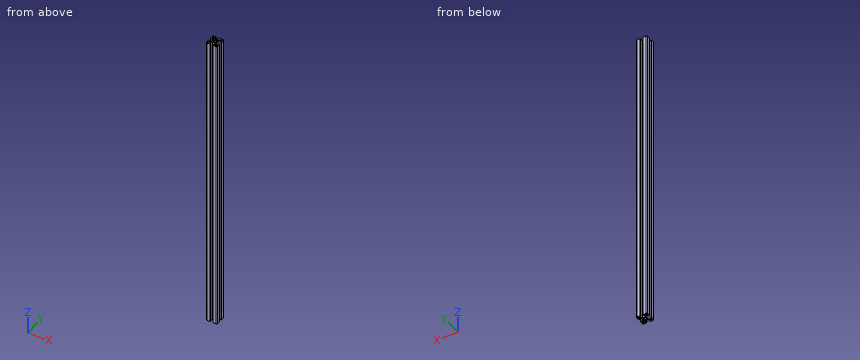
Autodesk Inventor part; units mm, degrees
ref_plane "YZ Plane" through (0, 0, 0) normal (1, 0, 0) x (0, 1, 0)
ref_plane "XZ Plane" through (0, 0, 0) normal (0, 1, 0) x (-1, 0, 0)
ref_plane "XY Plane" through (0, 0, 0) normal (0, 0, 1) x (1, 0, 0)
sketch "T-Slot 4040 Base" plane through (0, 0, 0) normal (0, 0, 1) x (1, 0, 0)
  line L0 (-28, 0) -> (28, 0) construction
  line L1 (0, -28) -> (0, 28) construction
  circle A0 centre (0, 0) radius 5.1
  line L2 (-7.5, -7.5) -> (7.5, -7.5)
  line L3 (7.5, -7.5) -> (7.5, 7.5)
  line L4 (7.5, 7.5) -> (-7.5, 7.5)
  line L5 (-7.5, 7.5) -> (-7.5, -7.5)
  line L6 (-7.5, -7.5) -> (7.5, 7.5) construction
  line L7 (7.5, -7.5) -> (-7.5, 7.5) construction
  line L8 (-20, 20) -> (20, 20)
  line L9 (20, 20) -> (20, -20)
  line L10 (20, -20) -> (-20, -20)
  line L11 (-20, -20) -> (-20, 20)
  line L12 (-20, 20) -> (20, -20) construction
  line L13 (20, 20) -> (-20, -20) construction
  line L14 (20, 5) -> (14.5, 5)
  line L15 (14.5, 5) -> (14.5, 10)
  line L16 (14.5, 10) -> (12.4749, 10)
  line L17 (12.4749, 10) -> (7.5, 5.0251)
  line L18 (5, 20) -> (5, 14.5)
  line L19 (5, 14.5) -> (10, 14.5)
  line L20 (10, 14.5) -> (10, 12.4749)
  line L21 (10, 12.4749) -> (5.0251, 7.5)
  line L22 (18.5, 18.5) -> (11.5, 18.5)
  line L23 (11.5, 18.5) -> (11.5, 11.5)
  line L24 (11.5, 11.5) -> (18.5, 11.5)
  line L25 (18.5, 11.5) -> (18.5, 18.5)
  line L26 (18.5, 18.5) -> (11.5, 11.5) construction
  line L27 (11.5, 18.5) -> (18.5, 11.5) construction
  line L28 (3.0732, 1.3088) -> (4.38, 2.6125) construction
  line L29 (5.905, 4.1338) -> (4.1393, 5.9037)
  line L30 (4.1393, 5.9037) -> (2.6122, 4.3802)
  line L31 (1.3075, 3.0787) -> (3.0732, 1.3088) construction
  line L32 (3.0732, 1.3088) -> (4.1393, 5.9037) construction
  line L33 (5.905, 4.1338) -> (1.3075, 3.0787) construction
  line L34 (4.38, 2.6125) -> (5.905, 4.1338)
  line L35 (2.6122, 4.3802) -> (1.3075, 3.0787) construction
  line L36 (-20, 5) -> (-14.5, 5)
  line L37 (-14.5, 5) -> (-14.5, 10)
  line L38 (-14.5, 10) -> (-12.4749, 10)
  line L39 (-12.4749, 10) -> (-7.5, 5.0251)
  line L40 (-5, 20) -> (-5, 14.5)
  line L41 (-5, 14.5) -> (-10, 14.5)
  line L42 (-10, 14.5) -> (-10, 12.4749)
  line L43 (-10, 12.4749) -> (-5.0251, 7.5)
  line L44 (-18.5, 18.5) -> (-11.5, 18.5)
  line L45 (-11.5, 18.5) -> (-11.5, 11.5)
  line L46 (-11.5, 11.5) -> (-18.5, 11.5)
  line L47 (-18.5, 11.5) -> (-18.5, 18.5)
  line L48 (-5.905, 4.1338) -> (-4.1393, 5.9037)
  line L49 (-4.1393, 5.9037) -> (-2.6122, 4.3802)
  line L50 (-4.38, 2.6125) -> (-5.905, 4.1338)
  line L51 (7.5, -7.5) -> (-7.5, -7.5)
  line L52 (20, -5) -> (14.5, -5)
  line L53 (14.5, -5) -> (14.5, -10)
  line L54 (14.5, -10) -> (12.4749, -10)
  line L55 (12.4749, -10) -> (7.5, -5.0251)
  line L56 (5, -20) -> (5, -14.5)
  line L57 (5, -14.5) -> (10, -14.5)
  line L58 (10, -14.5) -> (10, -12.4749)
  line L59 (10, -12.4749) -> (5.0251, -7.5)
  line L60 (18.5, -18.5) -> (11.5, -18.5)
  line L61 (11.5, -18.5) -> (11.5, -11.5)
  line L62 (11.5, -11.5) -> (18.5, -11.5)
  line L63 (18.5, -11.5) -> (18.5, -18.5)
  line L64 (18.5, -18.5) -> (11.5, -11.5) construction
  line L65 (11.5, -18.5) -> (18.5, -11.5) construction
  line L66 (3.0732, -1.3088) -> (4.38, -2.6125) construction
  line L67 (5.905, -4.1338) -> (4.1393, -5.9037)
  line L68 (4.1393, -5.9037) -> (2.6122, -4.3802)
  line L69 (1.3075, -3.0787) -> (3.0732, -1.3088) construction
  line L70 (3.0732, -1.3088) -> (4.1393, -5.9037) construction
  line L71 (5.905, -4.1338) -> (1.3075, -3.0787) construction
  line L72 (4.38, -2.6125) -> (5.905, -4.1338)
  line L73 (2.6122, -4.3802) -> (1.3075, -3.0787) construction
  line L74 (-4.38, -2.6125) -> (-5.905, -4.1338)
  line L75 (-4.1393, -5.9037) -> (-2.6122, -4.3802)
  line L76 (-5.905, -4.1338) -> (-4.1393, -5.9037)
  line L77 (-12.4749, -10) -> (-7.5, -5.0251)
  line L78 (-10, -12.4749) -> (-5.0251, -7.5)
  line L79 (-10, -14.5) -> (-10, -12.4749)
  line L80 (-5, -14.5) -> (-10, -14.5)
  line L81 (-5, -20) -> (-5, -14.5)
  line L82 (-18.5, -18.5) -> (-11.5, -18.5)
  line L83 (-11.5, -18.5) -> (-11.5, -11.5)
  line L84 (-11.5, -11.5) -> (-18.5, -11.5)
  line L85 (-18.5, -11.5) -> (-18.5, -18.5)
  line L86 (-14.5, -10) -> (-12.4749, -10)
  line L87 (-14.5, -5) -> (-14.5, -10)
  line L88 (-20, -5) -> (-14.5, -5)
  point P0 (15, 15)
  point P1 (3.6062, 3.6062)
  point P2 (3.6062, 3.6062)
  point P3 (15, -15)
  point P4 (3.6062, -3.6062)
  point P5 (3.6062, -3.6062)
  dimension "d9" = 10.2
  dimension "d12" = 40
  dimension "d13" = 40
  dimension "d14" = 5.5
  dimension "d15" = 15
  dimension "d16" = 7
  dimension "d17" = 10
  dimension "d20" = 1.75
  dimension "d21" = 7
  dimension "d22" = 2
  dimension "d29" = 1.5
  dimension "d30" = 2.5
extrude "Extrusion1" add sketch "T-Slot 4040 Base" along normal blind 1087 contours L5 L4 L3 L2 | L2 L78 L79 L80 L81 L10 L11 L88 L87 L86 L77 L5 | L2 L3 L55 L54 L53 L52 L9 L10 L56 L57 L58 L59 | L39 L38 L37 L36 L11 L8 L40 L41 L42 L43 L4 L5 | L3 L4 L21 L20 L19 L18 L8 L9 L14 L15 L16 L17
fillet "Rundung1" radius 1 16 edges at (11.5, 18.5, 543.5) (18.5, 18.5, 543.5) (18.5, 11.5, 543.5) (11.5, 11.5, 543.5) (-11.5, 18.5, 543.5) (-18.5, 18.5, 543.5) (-18.5, 11.5, 543.5) (-11.5, 11.5, 543.5) (-18.5, -11.5, 543.5) (-11.5, -11.5, 543.5) (-11.5, -18.5, 543.5) (-18.5, -18.5, 543.5) (11.5, -18.5, 543.5) (11.5, -11.5, 543.5) (18.5, -11.5, 543.5) (18.5, -18.5, 543.5)
fillet "Rundung2" radius 3 4 edges at (20, 20, 543.5) (20, -20, 543.5) (-20, -20, 543.5) (-20, 20, 543.5)
properties part number "T-SLOT 4040 B-Type 1087mm"
The model under review builds one solid part; all positions refer to its coordinate system, in mm. Coordinates: 2 decimals unless noted, no trailing zeros. Answer in a Markdown table with one row per item. Add a question column.
Item 1: Clearance check with flat-ended pins moving along their axes: pin 1 (3 mm diameter, centred on y = -4, z = 288.5, fed in from -X); pin 2 (8 mm diameter, centred on x = 0, z = 678, fed in from -Y). State where each tip first meets the part, or that it passes through.
Item 2: We need section A-A on z = 695. Give the number of separate pieces and of enclosed holes in the cut face, plus the area to 3 significant figures.
Item 3: To check wall thickness, follow probe 1 along Y at (x, z) = (12.5, 986); probe 2 along Y at (x, z) = (-0.5, 593.5); probe 3 along X at (y, z) = (-8.5, 683.5). State the ranges of each line that lie inside material, in increasing order.
Final values:
| question | item | result |
|---|---|---|
| 1 | pin 1 | stops at x = -20 |
| 1 | pin 2 | stops at y = -7.5 |
| 2 | separate pieces | 1 |
| 2 | enclosed holes | 5 |
| 2 | area | 616 mm2 |
| 3 | probe 1 | y = -20 to -18.5, -11.5 to -10, 10 to 11.5, 18.5 to 20 |
| 3 | probe 2 | y = -7.5 to -5.08, 5.08 to 7.5 |
| 3 | probe 3 | x = -20 to -14.5, -10.97 to -6.03, 6.03 to 10.97, 14.5 to 20 |
